Autodesk Inventor part; units mm, degrees
ref_plane "YZ Plane" through (0, 0, 0) normal (1, 0, 0) x (0, 1, 0)
ref_plane "XZ Plane" through (0, 0, 0) normal (0, 1, 0) x (-1, 0, 0)
ref_plane "XY Plane" through (0, 0, 0) normal (0, 0, 1) x (1, 0, 0)
sketch "Sketch1" plane through (0, 0, 0) normal (0, 0, 1) x (1, 0, 0)
  line L0 (0, 0) -> (0, 15)
  line L1 (0, 15) -> (9.7, 15)
  line L2 (9.7, 15) -> (9.7, 9.5314)
  line L3 (9.7, 9.5314) -> (11, 8.2314)
  line L4 (11, 8.2314) -> (11, 7.1)
  line L5 (11, 7.1) -> (10.3, 7.1)
  line L6 (10.3, 7.1) -> (10.3, 5.9)
  line L7 (10.3, 5.9) -> (11, 5.2)
  line L8 (11, 5.2) -> (11, 0)
  line L9 (11, 0) -> (0, 0)
  dimension "d0" = 11
  dimension "d1" = 15
  dimension "d2" = 135
  dimension "d5" = 9.7
  dimension "d6" = 1.2
  dimension "d7" = 0.7
  dimension "d8" = 0.8
  dimension "d9" = 7.9
  dimension "d11" = 0
extrude "Extrusion1" add sketch "Sketch1" along normal blind 0.7
fillet "Fillet1" radius 0.8 4 edges at (9.7, 15, 0.35) (0, 15, 0.35) (0, 0, 0.35) (11, 0, 0.35)
fillet "Fillet2" radius 0.4 3 edges at (9.7, 9.5314, 0.35) (11, 8.2314, 0.35) (10.3, 5.9, 0.35)
fillet "Fillet3" radius 0.2 1 edges at (10.3, 7.1, 0.35)
sketch "Sketch3" plane through (0, 0.8, 0) normal (-1, 0, 0) x (0, 0, 1)
  line L0 (0, 0) -> (0, 13.4)
  line L1 (0, 14.2) -> (0.3, 14.2)
  line L2 (0.3, 14.2) -> (0, 13.68)
  line L3 (0, 14.2) -> (0, 13.68)
  line L4 (0.7, 14.2) -> (0, 14.2)
  point P0 (0, -0.8)
  dimension "d17" = 0.52
  dimension "d18" = 0
  dimension "d19" = 0.3
extrude "Extrusion2" cut sketch "Sketch3" against normal through all
sketch "Sketch4" plane through (0, 0, 0.7) normal (0, 0, 1) x (1, 0, 0)
  line L0 (0, 0.8) -> (0, 14.2)
  arc A0 (0, 0.8) -> (0.8, 0) centre (0.8, 0.8) ccw
  line L1 (10.2, 0) -> (0.8, 0)
  arc A1 (10.2, 0) -> (11, 0.8) centre (10.2, 0.8) ccw
  line L2 (11, 5.2) -> (11, 0.8)
  arc A2 (11, 0.9915) -> (0, 0.9915) centre (5.5, -28.5) ccw
  point P0 (0, 0)
  dimension "d22" = 30
  dimension "d23" = 1.5
  dimension "d24" = 0.9915
  dimension "d25" = 0.9915
extrude "Extrusion3" add sketch "Sketch4" along normal blind 0.3
fillet "Fillet4" radius 0.2 2 edges at (5.5, 1.5, 0.7) (5.5, 1.5, 1)
equation "\"d24\" = d25"
Build history of the part. All positions in model axes, mm. Round coordinates to 2 decimals unless told otherwise and drop trailing zeros. Loops run counter-clockwise (first coordinate to the right, second up) from the corner with the lowest first, then second, coordinate; pieces in that order, holes last. Notation, with made-up numbers: (44.25, 63.5) -> (95.25, 63.5) arc R25 ccw to (95.25, 77.5) -> close; hole circle Ø9 at (-19.5, 4.25). An arc over 180 degrees is marked (long way). One line per item, written item: value. Start each with the question number.
Q1. Drop flat-ended pins along their axis: pin 1 Ø2 at (x, y) = (5, 4) entering from -Z; pin 2 Ø0.6 at (y, z) = (6.5, 0.5) entering from +X; pin 3 Ø3.5 at (x, y) = (5, 10) entering from +Z. Give the stop position or say it passes through.
Q2. Cut at B-B on y = 4. List the corners of the cut face in (x, z).
Q3. Cut at A-A on z = 0.55. List the corners of the cut face in (x, y), plus the area to 3 significant figures.
Q4. Probe line 1 along X through (y, z) = (10, 0.1); line 2 along X through (y, z) = (6.5, 0.15); line 3 along Z through (x, y) = (2.75, 13.75). List the from-to ranges inside material, lowest first.
Q5. Cut at C-C on y = 14. List the corners of the cut face in (x, z).
Computed:
1. pin 1: z = 0
1. pin 2: x = 10.3
1. pin 3: z = 0.7
2. outline: (0, 0) -> (11, 0) -> (11, 0.7) -> (0, 0.7) -> close
3. outline: (0, 0.8) arc R0.8 ccw to (0.8, 0) -> (10.2, 0) arc R0.8 ccw to (11, 0.8) -> (11, 5.2) -> (10.42, 5.78) arc R0.4 cw to (10.3, 6.07) -> (10.3, 6.9) arc R0.2 cw to (10.5, 7.1) -> (11, 7.1) -> (11, 8.07) arc R0.4 ccw to (10.88, 8.35) -> (9.82, 9.41) arc R0.4 cw to (9.7, 9.7) -> (9.7, 14.2) arc R0.8 ccw to (8.9, 15) -> (0.8, 15) arc R0.8 ccw to (0, 14.2) -> close
3. area: 155 mm²
4. line 1: 0 to 9.7
4. line 2: 0 to 10.3
4. line 3: 0 to 0.7
5. outline: (0, 0) -> (9.7, 0) -> (9.7, 0.7) -> (0, 0.7) -> close
